Here's how the part is built. I have some questions about the finished solid (model axes, mm). Face numbers are marked on the shaded views. A direction names the side the tool comes from. Give positions to 0.01 mm unless a question says otherwise; leave off trailing zeros. Order: outer loops, then holes, each group sorted by start corner. A loop starts at its lowest first (then second) coordinate and runs counter-clockwise, first axis right, second up. Notation, with made-up numbers: (56.5, 28) - (77.5, 28) arc R13 ccw to (77.5, 41) - close; hole circle Ø11 at (-36.5, 21.5). An arc over 180 degrees is marked (long way). One line per question, with ' | ' between items.
from build123d import *

# Parameters (mm, degrees)
BOSS_EXTRUDE1_DEPTH = 5
SKETCH3_R           = 1.5
CUT_EXTRUDE1_DEPTH  = 65.335060426


with BuildPart() as part:
    # Sketch1 → Boss-Extrude1 (new, symmetric)
    with BuildSketch(Plane.XY):
        Polygon((-55, 16.5), (-37, 16.5), (-32.015833371, 15.395447006), (32.015833371, 15.395447006), (37, 16.5), (55, 16.5), (55, -16.5), (37, -16.5), (32.015833371, -15.395447006), (-32.015833371, -15.395447006), (-37, -16.5), (-55, -16.5), align=None)
        with BuildLine():
            Line((-14.610208109, 4.550286626), (14.610208109, 4.550286626))
            ThreePointArc((14.610208109, 4.550286626), (23.186065182, 10.254148163), (24.151366397, 0))
            ThreePointArc((24.151366397, 0), (23.186065182, -10.254148163), (14.610208109, -4.550286626))
            Line((14.610208109, -4.550286626), (-14.610208109, -4.550286626))
            ThreePointArc((-14.610208109, -4.550286626), (-23.186065182, -10.254148163), (-24.151366397, 0))
            ThreePointArc((-24.151366397, 0), (-23.186065182, 10.254148163), (-14.610208109, 4.550286626))
        make_face(mode=Mode.SUBTRACT)
    extrude(amount=BOSS_EXTRUDE1_DEPTH, both=True)

    # Sketch3 → Cut-Extrude1 (cut, through all)
    with BuildSketch(Plane(origin=(0, 16.5, 0), x_dir=(1, 0, 0), z_dir=(0, 1, 0))):
        with Locations(Location((-50, 0, 0), (0, 0, 180))):
            Circle(SKETCH3_R)
        with Locations(Location((-43, 0, 0), (0, 0, 180))):
            Circle(SKETCH3_R)
        with Locations(Location((43, 0, 0), (0, 0, 180))):
            Circle(SKETCH3_R)
        with Locations(Location((50, 0, 0), (0, 0, 180))):
            Circle(SKETCH3_R)
    extrude(amount=-CUT_EXTRUDE1_DEPTH, mode=Mode.SUBTRACT)


solid = part.part
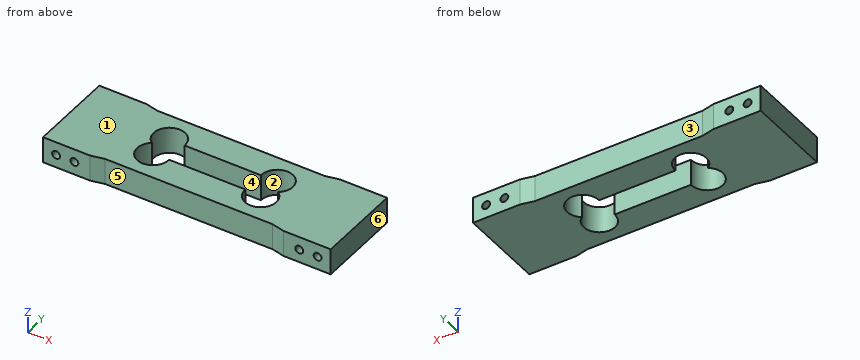
1) I want a section at B-B (y = 3). List the corners of the cut face in (x, z) for me.
Model answer:
outline: (-55, -5) - (-26.31, -5) - (-26.31, 5) - (-55, 5) - close; (26.31, -5) - (55, -5) - (55, 5) - (26.31, 5) - close; hole circle Ø3 at (-50, 0); hole circle Ø3 at (-43, 0); hole circle Ø3 at (43, 0); hole circle Ø3 at (50, 0)
2) I want a section at D-D (x = 43). List the corners of the cut face in (y, z) for me.
Model answer:
outline: (-16.5, -5) - (16.5, -5) - (16.5, -1.5) - (-16.5, -1.5) - close; (-16.5, 1.5) - (16.5, 1.5) - (16.5, 5) - (-16.5, 5) - close
3) I want a section at A-A (x = 1). List the corners of the cut face in (y, z) for me.
Model answer:
outline: (-15.4, -5) - (-4.55, -5) - (-4.55, 5) - (-15.4, 5) - close; (4.55, -5) - (15.4, -5) - (15.4, 5) - (4.55, 5) - close
4) Please list where these lines run through material, in increasing order: L1, parallel to Z at x = 50, y = 1; L2, parallel to X at y = -7.5, z = -3; L3, parallel to Y at x = -1, z = 2.
Model answer:
L1: z = -5 to -1.5, 1.5 to 5 | L2: x = -55 to -25.98, -15.23 to 15.23, 25.98 to 55 | L3: y = -15.4 to -4.55, 4.55 to 15.4
5) Thinking about a two-plate mould opening in Y: for the marked faces 1, 2 and 3, which applies, +Y half, -Y half, draft (parallel to the pull), parting line (faces both ways), or undercut?
Model answer:
face 1: draft | face 2: undercut | face 3: +Y half
6) On a 3-axis mill with a long thin cutter (end or side, diameter ignored), from which of +Z, -Z, +X, -X, +Y, -Y can I reach the whole of each face in a straight line? I mean the marked faces 4, 5 and 6. Say none if no direction works.
Model answer:
face 4: +Z, -Z | face 5: +Z, -Z, -Y | face 6: +Z, -Z, +X, +Y, -Y
7) I'm going to push flat-ended pins straight in: P1, Ø1, axis at x = -32.5, z = -3, coming from the -Y side; P2, Ø12, axis at x = -5.5, y = -1, coming from the -Z side; P3, Ø5, axis at x = 2, z = 1, coming from the -Y side; P4, Ø5, axis at x = -30, z = 3, coming from the -Y side. Where does each tip first touch, or does it pass through?
Model answer:
P1: stops at y = -15.61 | P2: stops at z = -5 | P3: stops at y = -15.4 | P4: stops at y = -15.5
8) I want a section at C-C (z = -3.25). List the corners of the cut face in (x, y) for me, plus the area to 3 significant figures.
Model answer:
outline: (-55, -16.5) - (-37, -16.5) - (-32.02, -15.4) - (32.02, -15.4) - (37, -16.5) - (55, -16.5) - (55, 16.5) - (37, 16.5) - (32.02, 15.4) - (-32.02, 15.4) - (-37, 16.5) - (-55, 16.5) - close; hole (-24.15, 0) arc R6 ccw (long way) to (-14.61, -4.55) - (14.61, -4.55) arc R6 ccw (long way) to (24.15, 0) arc R6 ccw (long way) to (14.61, 4.55) - (-14.61, 4.55) arc R6 ccw (long way) to start | area: 2,770 mm2
